Source: three-view drawing plus pictorial views. Frame: mm from the lowest corner of the part. A direction names the side the tool comes from. Give positions to 0.01 mm unless a question says otherwise; leave off trailing zeros. One line per item, written item: value.
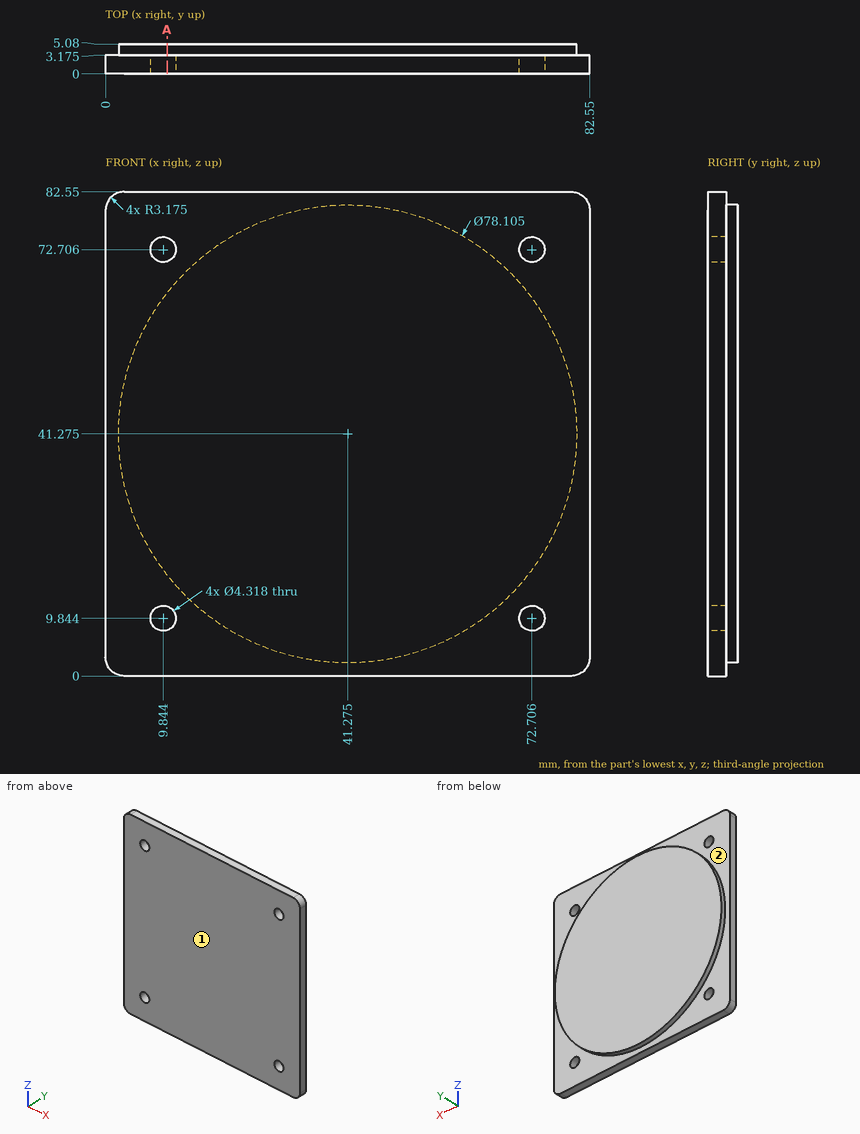
Item 1: Material intervals for L1, parallel to Y at x = 72, z = 75 (3 decimals); L2, parallel to Z at x = 65, y = 4.85 (1 decimal); L3, parallel to Z at x = 67.5, y = 3.8, sorted ascending.
Verdict:
L1: y = 0 to 3.175
L2: z = 10.3 to 72.3
L3: z = 12.34 to 70.21
Item 2: Pin query (flat end, axial travel): P1, Ø1, axis at x = 8.5, y = 4, coming from the -Z side. Return the tip coordinate at first contact, or that it passes through.
Verdict:
P1: stops at z = 19.29
Item 3: Access query for the marked faces 1 and 2. Directions: +Z, -Z, +X, -X, +Y, -Y. A direction counts if a zero-diameter tool reaches every point of the face in a straight line with its end or side. Return the directions, or none.
Verdict:
face 1: +Z, -Z, +X, -X, -Y
face 2: +Y
Item 4: Section A-A, the plane x = 10.5. Count the separate pieces of the cut face and the enclosed holes in it, and give its area (3 significant figures).
Verdict:
separate pieces: 3
enclosed holes: 0
area: 328 mm^2
